Model file for the job. Use its own axes, mm. A direction names the side the tool comes from. Coordinates: 2 decimals unless noted, no trailing zeros. Order: outer loops, then holes, each group sorted by start corner. A loop starts at its lowest first (then second) coordinate and runs counter-clockwise, first axis right, second up. Notation, with made-up numbers: (-20.5, 11) -> (21.5, 11) arc R23 cw to (21.5, 44) -> close; hole circle Ø1 at (-21.75, -2). An arc over 180 degrees is marked (long way). Write item = value, one per line. Start each with the question number.
Q1. Wall check: line 1 (Z direction, x = 132.5, y = 87.5); line 2 (X direction, y = 102, z = 18.75); line 3 (X direction, y = 24, z = 19). Give the ranges that are in metal, low to high. Write a range as from..to.
Q2. Mould opens along Y. For faces 1 (the face through (103.421, 19.256, 16.457)), 2 (the face through (76, 23, 20.32)) say: +Y half, -Y half, draft (parallel to the pull), parting line (faces both ways), or undercut.
Q3. Cut at D-D, the plane y = 24.5. List the corners of the cut face in (x, z), plus the area to 3 significant figures.
Q4. 3-axis set-ups, long thin cutter, end or side, ignore diameter. For faces 3 (the face through (24.35, 76.99, 16.46)), 4 (the face through (101, 48, 20.32)): which of +Z, -Z, +X, -X, +Y, -Y reach the whole face in a straight line?
Q5. Cut at B-B, the plane x = 100. List the corners of the cut face in (y, z), plus the area to 3 significant figures.
Q6. Cut at C-C, the plane y = 67. List the corners of the cut face in (x, z), plus the area to 3 significant figures.
Q7. Cut at A-A, the plane z = 18. Give the number of separate pieces and of enclosed holes in the cut face, plus the area to 3 significant figures.
Autodesk Inventor part; units mm, degrees
ref_plane "YZ Plane" through (0, 0, 0) normal (1, 0, 0) x (0, 1, 0)
ref_plane "XZ Plane" through (0, 0, 0) normal (0, 1, 0) x (-1, 0, 0)
ref_plane "XY Plane" through (0, 0, 0) normal (0, 0, 1) x (1, 0, 0)
sketch "Sketch1" plane through (0, 0, 0) normal (0, 0, 1) x (1, 0, 0)
  line L0 (12.4728, 9.7682) -> (164.8728, 9.7682)
  line L1 (164.8728, 9.7682) -> (164.8728, 111.3682)
  line L2 (164.8728, 111.3682) -> (12.4728, 111.3682)
  line L3 (12.4728, 111.3682) -> (12.4728, 9.7682)
  point P0 (0, 0)
  dimension "d0" = 152.4
  dimension "d1" = 101.6
extrude "Extrusion1" add sketch "Sketch1" along normal blind 12.7
sketch "Sketch2" plane through (0, 0, 12.7) normal (0, 0, 1) x (1, 0, 0)
  circle A0 centre (25.1728, 22.4682) radius 3.81
  line L0 (12.4728, 111.3682) -> (12.4728, 9.7682)
  line L1 (12.4728, 9.7682) -> (164.8728, 9.7682)
  circle A1 centre (25.1728, 47.8682) radius 3.81
  circle A2 centre (25.1728, 73.2682) radius 3.81
  circle A3 centre (25.1728, 98.6682) radius 3.81
  circle A4 centre (50.5728, 22.4682) radius 3.81
  circle A5 centre (50.5728, 47.8682) radius 3.81
  circle A6 centre (50.5728, 73.2682) radius 3.81
  circle A7 centre (50.5728, 98.6682) radius 3.81
  circle A8 centre (75.9728, 22.4682) radius 3.81
  circle A9 centre (75.9728, 47.8682) radius 3.81
  circle A10 centre (75.9728, 73.2682) radius 3.81
  circle A11 centre (75.9728, 98.6682) radius 3.81
  circle A12 centre (101.3728, 22.4682) radius 3.81
  circle A13 centre (101.3728, 47.8682) radius 3.81
  circle A14 centre (101.3728, 73.2682) radius 3.81
  circle A15 centre (101.3728, 98.6682) radius 3.81
  circle A16 centre (126.7728, 22.4682) radius 3.81
  circle A17 centre (126.7728, 47.8682) radius 3.81
  circle A18 centre (126.7728, 73.2682) radius 3.81
  circle A19 centre (126.7728, 98.6682) radius 3.81
  circle A20 centre (152.1728, 22.4682) radius 3.81
  circle A21 centre (152.1728, 47.8682) radius 3.81
  circle A22 centre (152.1728, 73.2682) radius 3.81
  circle A23 centre (152.1728, 98.6682) radius 3.81
  point P0 (0, 0)
  dimension "d4" = 7.62
  dimension "d5" = 12.7
  dimension "d6" = 12.7
  dimension "d9" = 25.4
  dimension "d12" = 25.4
extrude "Extrusion2" add sketch "Sketch2" along normal blind 7.62
properties part number "p"
Here are the results:
q1.line_1 = 0..12.7
q1.line_2 = 23.32..27.02, 48.72..52.42, 74.12..77.82, 99.52..103.22, 124.92..128.62, 150.32..154.02
q1.line_3 = 21.68..28.66, 47.08..54.06, 72.48..79.46, 97.88..104.86, 123.28..130.26, 148.68..155.66
q2.face_1 = undercut
q2.face_2 = draft
q3.outline = (12.47, 0) -> (164.87, 0) -> (164.87, 12.7) -> (155.4, 12.7) -> (155.4, 20.32) -> (148.95, 20.32) -> (148.95, 12.7) -> (130, 12.7) -> (130, 20.32) -> (123.55, 20.32) -> (123.55, 12.7) -> (104.6, 12.7) -> (104.6, 20.32) -> (98.15, 20.32) -> (98.15, 12.7) -> (79.2, 12.7) -> (79.2, 20.32) -> (72.75, 20.32) -> (72.75, 12.7) -> (53.8, 12.7) -> (53.8, 20.32) -> (47.35, 20.32) -> (47.35, 12.7) -> (28.4, 12.7) -> (28.4, 20.32) -> (21.95, 20.32) -> (21.95, 12.7) -> (12.47, 12.7) -> close
q3.area = 2,230 mm²
q4.face_3 = +Z
q4.face_4 = +Z, +X, -X, +Y, -Y
q5.outline = (9.77, 0) -> (111.37, 0) -> (111.37, 12.7) -> (102.22, 12.7) -> (102.22, 20.32) -> (95.11, 20.32) -> (95.11, 12.7) -> (76.82, 12.7) -> (76.82, 20.32) -> (69.71, 20.32) -> (69.71, 12.7) -> (51.42, 12.7) -> (51.42, 20.32) -> (44.31, 20.32) -> (44.31, 12.7) -> (26.02, 12.7) -> (26.02, 20.32) -> (18.91, 20.32) -> (18.91, 12.7) -> (9.77, 12.7) -> close
q5.area = 1,510 mm²
q6.outline = (12.47, 0) -> (164.87, 0) -> (164.87, 12.7) -> (12.47, 12.7) -> close
q6.area = 1,940 mm²
q7.separate_pieces = 24
q7.enclosed_holes = 0
q7.area = 1,090 mm²
